Geometry check sheet. Reference: the model listing, model coordinates, mm. A direction names the side the tool comes from. Round coordinates to 2 decimals unless told otherwise and drop trailing zeros. Write each loop counter-clockwise with the first axis right and the second up, starting at its lowest first coordinate (ties: lowest second). Pieces come first, ordered by that corner, then holes. Notation, with made-up numbers: (20.5, -1.75) -> (79.5, -1.75) arc R21 cw to (79.5, 21.25) -> close; hole circle Ø3 at (-36.75, -10). An arc over 180 degrees is marked (long way). Use a Markdown table: item, result.
```python
from build123d import *

# Parameters (mm, degrees)
SKETCH1_R           = 21.1
SKETCH1_R_2         = 18.6
BOSS_EXTRUDE4_DEPTH = 58.8
SKETCH4_R           = 21.1
BOSS_EXTRUDE5_DEPTH = 2.5
SKETCH12_W          = 42.2
SKETCH12_H          = 42.2
BOSS_EXTRUDE6_DEPTH = 42.2
SKETCH13_R          = 21.1
BOSS_EXTRUDE7_DEPTH = 350
CUT_EXTRUDE1_DEPTH  = 21.5
SKETCH15_R          = 3
CUT_EXTRUDE2_DEPTH  = 9.5
SKETCH16_R          = 6.025
CUT_EXTRUDE3_DEPTH  = 6.2
SKETCH17_W          = 37.2
SKETCH17_H          = 37.2
CUT_EXTRUDE4_DEPTH  = 39.7
SKETCH18_R          = 15
CUT_EXTRUDE5_DEPTH  = 5
SKETCH19_R          = 1.827460326
CUT_EXTRUDE6_DEPTH  = 2.5
SKETCH23_R          = 17.945895708
CUT_EXTRUDE7_DEPTH  = 2.5


with BuildPart() as part:
    # Sketch1 → Boss-Extrude4 (new body)
    with BuildSketch(Plane.XY):
        Circle(SKETCH1_R)
        Circle(SKETCH1_R_2, mode=Mode.SUBTRACT)
    extrude(amount=BOSS_EXTRUDE4_DEPTH)

    # Sketch4 → Boss-Extrude5 (add)
    with BuildSketch(Plane(origin=(0, 0, 0), x_dir=(-1, 0, 0), z_dir=(0, 0, -1))):
        Circle(SKETCH4_R)
    extrude(amount=BOSS_EXTRUDE5_DEPTH)

    # Sketch12 → Boss-Extrude6 (add)
    with BuildSketch(Plane(origin=(0, 0, -2.5), x_dir=(-1, 0, 0), z_dir=(0, 0, -1))):
        Rectangle(SKETCH12_W, SKETCH12_H)
    extrude(amount=BOSS_EXTRUDE6_DEPTH)

    # Sketch13 → Boss-Extrude7 (add)
    with BuildSketch(Plane(origin=(0, -21.1, 0), x_dir=(-1, 0, 0), z_dir=(0, -1, 0))):
        with Locations((0, 23.6)):
            Circle(SKETCH13_R)
    extrude(amount=BOSS_EXTRUDE7_DEPTH)

    # Sketch14 → Cut-Extrude1 (cut)
    with BuildSketch(Plane(origin=(0, -371.1, 0), x_dir=(-1, 0, 0), z_dir=(0, -1, 0))):
        with BuildLine():
            Line((-1.68529671, 21.1), (1.68529671, 21.1))
            ThreePointArc((1.68529671, 21.1), (0, 26.615), (-1.68529671, 21.1))
        make_face()
    extrude(amount=-CUT_EXTRUDE1_DEPTH, mode=Mode.SUBTRACT)

    # Sketch15 → Cut-Extrude2 (cut)
    with BuildSketch(Plane(origin=(0, -371.1, 0), x_dir=(-1, 0, 0), z_dir=(0, -1, 0))):
        with Locations((0, 23.6)):
            Circle(SKETCH15_R)
    extrude(amount=-CUT_EXTRUDE2_DEPTH, mode=Mode.SUBTRACT)

    # Sketch16 → Cut-Extrude3 (cut)
    with BuildSketch(Plane(origin=(0, -371.1, 0), x_dir=(-1, 0, 0), z_dir=(0, -1, 0))):
        with Locations((0, 23.6)):
            Circle(SKETCH16_R)
    extrude(amount=-CUT_EXTRUDE3_DEPTH, mode=Mode.SUBTRACT)

    # Sketch17 → Cut-Extrude4 (cut)
    with BuildSketch(Plane(origin=(0, 0, -44.7), x_dir=(-1, 0, 0), z_dir=(0, 0, -1))):
        Rectangle(SKETCH17_W, SKETCH17_H)
    extrude(amount=-CUT_EXTRUDE4_DEPTH, mode=Mode.SUBTRACT)

    # Sketch18 → Cut-Extrude5 (cut)
    with BuildSketch(Plane.XY):
        Circle(SKETCH18_R)
    extrude(amount=-CUT_EXTRUDE5_DEPTH, mode=Mode.SUBTRACT)

    # Sketch19 → Cut-Extrude6 (cut)
    with BuildSketch(Plane(origin=(0, -21.1, 0), x_dir=(-1, 0, 0), z_dir=(0, -1, 0))):
        with Locations((-16.772539674, 40.372539674)):
            Circle(SKETCH19_R)
    extrude(amount=-CUT_EXTRUDE6_DEPTH, mode=Mode.SUBTRACT)

    # Sketch23 → Cut-Extrude7 (cut)
    with BuildSketch(Plane(origin=(0, -21.1, 0), x_dir=(-1, 0, 0), z_dir=(0, -1, 0))):
        with Locations((-0.654104292, 23.6)):
            Circle(SKETCH23_R)
    extrude(amount=-CUT_EXTRUDE7_DEPTH, mode=Mode.SUBTRACT)


solid = part.part
```
(1) Section check A-A on z = -33. Record the cut outline in (x, y), plus the area to 3 significant figures.
A:
| item | result |
|---|---|
| outline | (-21.1, -21.1) -> (-18.89, -21.1) -> (-18.89, -371.1) -> (18.89, -371.1) -> (18.89, -21.1) -> (21.1, -21.1) -> (21.1, 21.1) -> (-21.1, 21.1) -> close; hole (-18.6, -18.6) -> (-14.63, -18.6) -> (-14.63, -21.1) -> (15.94, -21.1) -> (15.94, -18.6) -> (18.6, -18.6) -> (18.6, 18.6) -> (-18.6, 18.6) -> close |
| area | 13,500 mm2 |
(2) Section check D-D on z = 34. Record the cut outline in (x, y).
A:
| item | result |
|---|---|
| outline | circle Ø42.2 at (0, 0); hole circle Ø37.2 at (0, 0) |
(3) Access from +Z, -Z, +X, -X, +Y, -Y to the whole of each face (thin tool, end or side, straight path). Record for faces 4 (the face through (13.88, -19.87, -35.73)), 5 (the face through (17, 16, -2.5)), 6 (the face through (-16, -21.1, -7)).
A:
| item | result |
|---|---|
| face 4 | none |
| face 5 | +Z, +X, +Y |
| face 6 | +Z, -X, -Y |
(4) Section check C-C on y = -105. Record the cut outline in (x, z).
A:
| item | result |
|---|---|
| outline | circle Ø42.2 at (0, -23.6) |
(5) Release check for a two-part mould opening along X. For faces 1 (the face through (4.57, -193.65, -3)), 2 (the face through (0, -19, 58.8)), 3 (the face through (-14.985, 0.66, -2.465)) record: +X half, -X half, draft (parallel to the pull), parting line (faces both ways), or undercut.
A:
| item | result |
|---|---|
| face 1 | parting line |
| face 2 | draft |
| face 3 | undercut |
(6) Section check B-B on x = -9.5. Record the cut outline in (y, z), plus the area to 3 significant figures.
A:
| item | result |
|---|---|
| outline | (-371.1, -42.44) -> (-21.1, -42.44) -> (-21.1, -44.7) -> (-18.6, -44.7) -> (-18.6, -38.4) -> (-21.1, -38.4) -> (-21.1, -8.8) -> (-18.6, -8.8) -> (-18.6, -5) -> (-11.61, -5) -> (-11.61, 0) -> (-15.99, 0) -> (-15.99, 58.8) -> (-18.84, 58.8) -> (-18.84, -2.5) -> (-21.1, -2.5) -> (-21.1, -4.76) -> (-371.1, -4.76) -> close; (11.61, -5) -> (18.6, -5) -> (18.6, -44.7) -> (21.1, -44.7) -> (21.1, -2.5) -> (18.84, -2.5) -> (18.84, 58.8) -> (15.99, 58.8) -> (15.99, 0) -> (11.61, 0) -> close |
| area | 13,700 mm2 |
(7) Gauge pin test, flat ends, axial feed: pin 1 Ø1 at (x, z) = (-12, -1) entering from -Y; pin 2 Ø12 at (x, y) = (-7.5, -182) entering from -Z; pin 3 Ø3 at (x, z) = (16.77, -40.37) entering from -Y. Record the tip position at first contact, or that the pin passes through.
A:
| item | result |
|---|---|
| pin 1 | stops at y = -17.69 |
| pin 2 | stops at z = -44.65 |
| pin 3 | stops at y = 18.6 |
(8) Thickness scan on line 1 (Y direction, x = 0, z = 22); line 2 (X direction, y = -355, z = -23); line 3 (X direction, y = -20, z = -23). Record the ranges inside material, lowest first.
A:
| item | result |
|---|---|
| line 1 | y = -21.1 to -18.6, 18.6 to 21.1 |
| line 2 | x = -21.09 to -2.95, 2.95 to 21.09 |
| line 3 | x = -21.1 to -17.28, 18.59 to 21.1 |
